Source: CAD feature listing. Evaluate the final solid. Frame: model axes, mm. A direction names the side the tool comes from. Round coordinates to 2 decimals unless told otherwise and drop trailing zeros. Order: outer loops, then holes, each group sorted by start corner. A loop starts at its lowest first (then second) coordinate and runs counter-clockwise, first axis right, second up. Notation, with made-up numbers: (65, 49.25) -> (70, 49.25) arc R30 ccw to (70, 75.25) -> close; hole circle Ø8 at (82.25, -29). An arc over 180 degrees is marked (long way). One line per item, written item: value. Start each with the question number.
1) Reachability of faces 4 (the face through (31.954, -4, 15)), 5 (the face through (-44.354, -4, 15)), 6 (the face through (-38, -5.892, 15)) from +Z, -Z, +X, -X, +Y, -Y: full face, straight path, thin tool, end or side. Return the list, or none.
2) Ray query, L1, parallel to Y at x = -53, z = 1.8; L2, parallel to Z at x = -47.5, y = -2.25; L3, parallel to Y at x = -34, z = 14.5. Return the intervals inside material, ascending.
3) Pin query (flat end, axial travel): P1, Ø3.5, axis at x = -38.154, z = 18.297, coming from the -Y side; P2, Ø6, axis at x = 37, z = 11, coming from the -Y side; P3, Ø10, axis at x = -35.5, z = 17, coming from the +Y side; P4, Ø2, axis at y = -3.5, z = 14, coming from the -X side. Return the tip coordinate at first contact, or that it passes through.
4) Section B-B (z = 11.75). Return the cut outline in (x, y), and give its area (3 significant figures).
5) Mould query, pull axis X, two halves, no side actions, for faces 1 (the face through (44.354, -4, 15)), 2 (the face through (-55.2, 0.8, 2)), 3 (the face through (-38.03, -6.79, 3.86)). Classes: pulls with the +X half, pulls with the -X half, needs draft (parallel to the pull), parting line crosses it, or undercut.
6) Section A-A (x = 53). Return the cut outline in (y, z), and give its area (3 significant figures).
7) Section D-D (x = -22). Return the cut outline in (y, z), and give its area (3 significant figures).
8) Section C-C (z = 17.25). Return the cut outline in (x, y).
```python
from build123d import *

# Parameters (mm, degrees)
SKETCH_W     = 126
SKETCH_H     = 25
SKETCH_R     = 2.2
PAD_DEPTH    = 3
SKETCH001_W  = 12.4
SKETCH001_H  = 4
PAD001_DEPTH = 21.497
SKETCH002_R  = 2.2
POCKET_DEPTH = 4
CHAMFER_SIZE = 1
FILLET_R     = 3


with BuildPart() as part:
    # Sketch → Pad (new body)
    with BuildSketch(Plane.XY):
        Rectangle(SKETCH_W, SKETCH_H)
        with Locations((-53, 0.726)):
            Circle(SKETCH_R, mode=Mode.SUBTRACT)
        with Locations((53, 0.726)):
            Circle(SKETCH_R, mode=Mode.SUBTRACT)
    extrude(amount=PAD_DEPTH)

    # Sketch001 → Pad001 (new body)
    with BuildSketch(Plane.XY.offset(3)):
        with Locations((-38.154, -3.892)):
            Rectangle(SKETCH001_W, SKETCH001_H)
        with Locations((38.154, -3.892)):
            Rectangle(SKETCH001_W, SKETCH001_H)
    extrude(amount=PAD001_DEPTH)

    # Sketch002 → Pocket (cut)
    with BuildSketch(Plane.XZ.offset(5.892)):
        with Locations((-38.154, 18.297)):
            Circle(SKETCH002_R)
    pocket = extrude(amount=-POCKET_DEPTH, mode=Mode.SUBTRACT)

    # Mirrored: Pocket across Sketch002 V_Axis
    add(pocket.mirror(Plane(origin=(0, -5.892, 0), x_dir=(0, -1, 0), z_dir=(1, 0, 0))), mode=Mode.SUBTRACT)

    # Chamfer
    chamfer_edges = [part.edges().sort_by_distance(p)[0] for p in [
        (0, 12.5, 0),
        (63, 0, 0),
        (0, -12.5, 0),
        (-63, 0, 0),
        (50.8, 0.726, 0),
        (-55.2, 0.726, 0),
    ]]
    chamfer(chamfer_edges, length=CHAMFER_SIZE)

    # Fillet
    fillet_edges = [part.edges().sort_by_distance(p)[0] for p in [
        (38.154, -5.892, 3),
        (31.954, -3.892, 3),
        (38.154, -1.892, 3),
        (44.354, -3.892, 3),
        (-38.154, -5.892, 3),
        (-31.954, -3.892, 3),
        (-38.154, -1.892, 3),
        (-44.354, -3.892, 3),
    ]]
    fillet(fillet_edges, radius=FILLET_R)


solid = part.part
```
Findings:
1. face 4: +Z, +Y, -Y
1. face 5: +Z, -X, +Y, -Y
1. face 6: +Z, +X, -X, -Y
2. L1: -12.5 to -1.47, 2.93 to 12.5
2. L2: 0 to 3
2. L3: -5.89 to -1.89
3. P1: through
3. P2: y = -5.89
3. P3: y = -1.89
3. P4: x = -44.35
4. outline: (-44.35, -5.89) -> (-31.95, -5.89) -> (-31.95, -1.89) -> (-44.35, -1.89) -> close; (31.95, -5.89) -> (44.35, -5.89) -> (44.35, -1.89) -> (31.95, -1.89) -> close
4. area: 99.2 mm2
5. face 1: pulls with the +X half
5. face 2: undercut
5. face 3: needs draft
6. outline: (-12.5, 1) -> (-11.5, 0) -> (-2.47, 0) -> (-1.47, 1) -> (-1.47, 3) -> (-12.5, 3) -> close; (2.93, 1) -> (3.93, 0) -> (11.5, 0) -> (12.5, 1) -> (12.5, 3) -> (2.93, 3) -> close
6. area: 59.8 mm2
7. outline: (-12.5, 1) -> (-11.5, 0) -> (11.5, 0) -> (12.5, 1) -> (12.5, 3) -> (-12.5, 3) -> close
7. area: 74.0 mm2
8. outline: (-44.35, -5.89) -> (-40.09, -5.89) -> (-40.09, -1.89) -> (-44.35, -1.89) -> close; (-36.22, -5.89) -> (-31.95, -5.89) -> (-31.95, -1.89) -> (-36.22, -1.89) -> close; (31.95, -5.89) -> (36.22, -5.89) -> (36.22, -1.89) -> (31.95, -1.89) -> close; (40.09, -5.89) -> (44.35, -5.89) -> (44.35, -1.89) -> (40.09, -1.89) -> close
